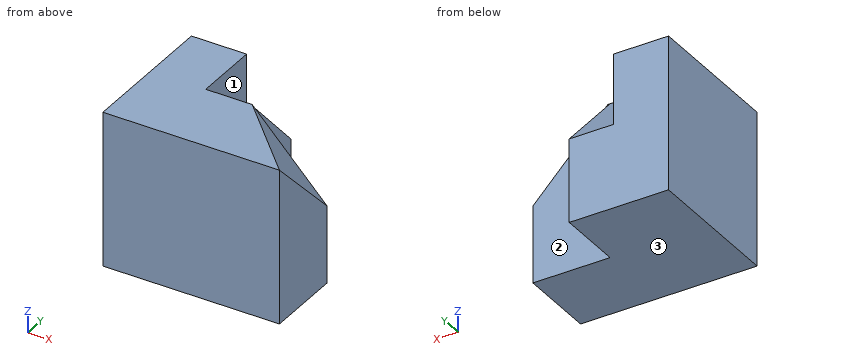
```python
from build123d import *

# Parameters (mm, degrees)
CROQUIS1_W              = 80
CROQUIS1_H              = 70
SALIENTE_EXTRUIR1_DEPTH = 65
CROQUIS2_W              = 70
CROQUIS2_H              = 30
CORTAR_EXTRUIR1_DEPTH   = 35
CORTAR_EXTRUIR2_DEPTH   = 20
CORTAR_EXTRUIR3_DEPTH   = 20


with BuildPart() as part:
    # Croquis1 → Saliente-Extruir1 (new body)
    with BuildSketch(Plane(origin=(0, 0, 0), x_dir=(1, 0, 0), z_dir=(0, 1, 0))):
        with Locations((40, 35)):
            Rectangle(CROQUIS1_W, CROQUIS1_H)
    extrude(amount=SALIENTE_EXTRUIR1_DEPTH)

    # Croquis2 → Cortar-Extruir1 (cut)
    with BuildSketch(Plane(origin=(80, 0, 0), x_dir=(0, 0, -1), z_dir=(1, 0, 0))):
        with Locations((35, 50)):
            Rectangle(CROQUIS2_W, CROQUIS2_H)
    extrude(amount=-CORTAR_EXTRUIR1_DEPTH, mode=Mode.SUBTRACT)

    # Croquis3 → Cortar-Extruir2 (cut)
    with BuildSketch(Plane(origin=(45, 0, 0), x_dir=(0, 0, -1), z_dir=(1, 0, 0))):
        Polygon((0, 35), (32, 65), (0, 65), align=None)
    extrude(amount=-CORTAR_EXTRUIR2_DEPTH, mode=Mode.SUBTRACT)

    # Croquis6 → Cortar-Extruir3 (cut)
    with BuildSketch(Plane(origin=(27.763221793, 26.928249656, 26.928249656), x_dir=(0.4101501227910038, 0.39781495770089986, -0.8206827256644043), z_dir=(0.5891012412208205, 0.5713841648103704, 0.5713841648103701))):
        Polygon((32.812009823, -55.698422491), (75.459428741, -30.574775071), (32.812009823, -6.939578699), align=None)
    extrude(amount=CORTAR_EXTRUIR3_DEPTH, mode=Mode.SUBTRACT)


solid = part.part
```
Here's how the part is built. I have some questions about the finished solid (model axes, mm). Face numbers are marked on the shaded views. A direction names the side the tool comes from. Round coordinates to 2 decimals unless told otherwise and drop trailing zeros. Order: outer loops, then holes, each group sorted by start corner. A loop starts at its lowest first (then second) coordinate and runs counter-clockwise, first axis right, second up. Notation, with made-up numbers: M 44,82.5 L 82,82.5 A4 ccw 82,86.5 Z; hole C -17,47 d8. An arc over 180 degrees is marked long. Answer in a Markdown table with one row per item.
Item 1: Imagine slicing it at D-D, the plane x = 68.5. Write out the boundary of the cut face in (y, z).
A:
| item | result |
|---|---|
| outline | M 0,-70 L 35,-70 L 35,-23.14 L 11.86,0 L 0,0 Z |
Item 2: I'm going to push flat-ended pins straight in: pin 1 (1 mm diameter, centred on x = 26, y = 50, fed in from +Z); pin 2 (10 mm diameter, centred on y = 7.5, z = -60.5, fed in from -X); pin 3 (2 mm diameter, centred on y = 47.5, z = -59, fed in from +X); pin 4 (17.5 mm diameter, centred on x = 59.5, z = -49, fed in from +Y). Where does each tip first touch, or does it pass through?
A:
| item | result |
|---|---|
| pin 1 | stops at z = -15.47 |
| pin 2 | stops at x = 0 |
| pin 3 | stops at x = 45 |
| pin 4 | stops at y = 35 |
Item 3: Imagine slicing it at A-A, the plane y = 44. Write out the boundary of the cut face in (x, z), and give its area (3 significant figures).
A:
| item | result |
|---|---|
| outline | M 0,-70 L 45,-70 L 45,-9.6 L 25,-9.6 L 25,0 L 0,0 Z |
| area | 2,960 mm2 |
Item 4: Imagine slicing it at B-B, the plane x = 26.5. Write out the boundary of the cut face in (y, z), and give its area (3 significant figures).
A:
| item | result |
|---|---|
| outline | M 0,-70 L 65,-70 L 65,-32 L 35,0 L 0,0 Z |
| area | 4,070 mm2 |
Item 5: For the marked faces 1, 2 and 3, which set-ups out of +Z, -Z, +X, -X, +Y, -Y let a thin tool reach every point of the face, with its end or its side?
A:
| item | result |
|---|---|
| face 1 | +Z, +X, +Y |
| face 2 | +Z, -Z, +X, +Y |
| face 3 | -Z, +X, -X, +Y, -Y |
Item 6: Imagine slicing it at C-C, the plane z = -36.5. Write out the boundary of the cut face in (x, y), and give its area (3 significant figures).
A:
| item | result |
|---|---|
| outline | M 0,0 L 80,0 L 80,35 L 45,35 L 45,65 L 0,65 Z |
| area | 4,150 mm2 |
Item 7: If I drill on L1, parallel to Y at x = 68, z = -63.5; L2, parallel to X at y = 60, z = -29.5; L3, parallel to Y at x = 60.5, z = -11.5, over which ranges is the centre line in solid material (lowest first)? Write a range as from..to.
A:
| item | result |
|---|---|
| L1 | y = 0..35 |
| L2 | x = 0..45 |
| L3 | y = 0..31.6 |
